```python
from build123d import *

# Parameters (mm, degrees)
SKETCH1_R           = 3.5
SKETCH1_R_2         = 1.5
SKETCH1_R_3         = 2.5
SKETCH1_W           = 2
SKETCH1_H           = 5
SKETCH1_W_2         = 5.5
SKETCH1_H_2         = 15.95
SKETCH1_H_3         = 14.5
BOSS_EXTRUDE1_DEPTH = 2
CUT_EXTRUDE_1_DEPTH = 10


with BuildPart() as part:
    # Sketch1 → Boss-Extrude1 (new body)
    with BuildSketch(Plane.XY):
        with BuildLine():
            Line((-25.65, 0), (25.65, 0))
            ThreePointArc((25.65, 0), (26.357106781, 0.292893219), (26.65, 1))
            Line((26.65, 1), (26.65, 99.754415082))
            ThreePointArc((26.65, 99.754415082), (25.980127019, 102.254415082), (24.15, 104.0845421))
            Line((24.15, 104.0845421), (7.5, 113.697424082))
            ThreePointArc((7.5, 113.697424082), (0, 115.707043026), (-7.5, 113.697424082))
            Line((-7.5, 113.697424082), (-24.15, 104.0845421))
            ThreePointArc((-24.15, 104.0845421), (-25.980127019, 102.254415082), (-26.65, 99.754415082))
            Line((-26.65, 99.754415082), (-26.65, 1))
            ThreePointArc((-26.65, 1), (-26.357106781, 0.292893219), (-25.65, 0))
        make_face()
        with Locations((0, 90)):
            Circle(SKETCH1_R, mode=Mode.SUBTRACT)
        with Locations((19.05, 66.1)):
            Circle(SKETCH1_R_2, mode=Mode.SUBTRACT)
        with Locations((-8.85, 66.1)):
            Circle(SKETCH1_R_2, mode=Mode.SUBTRACT)
        with Locations((-24.05, 15.3)):
            Circle(SKETCH1_R_2, mode=Mode.SUBTRACT)
        with Locations((24.15, 14)):
            Circle(SKETCH1_R_2, mode=Mode.SUBTRACT)
        with Locations((0, 34.3)):
            Circle(SKETCH1_R_3, mode=Mode.SUBTRACT)
        with Locations((4.5, 103.75)):
            Rectangle(SKETCH1_W, SKETCH1_H, mode=Mode.SUBTRACT)
        with Locations((9.55, 83.375)):
            Rectangle(SKETCH1_W_2, SKETCH1_H_2, mode=Mode.SUBTRACT)
        with Locations((20.15, 87)):
            Rectangle(SKETCH1_W, SKETCH1_H_3, mode=Mode.SUBTRACT)
        with Locations((4.5, 72.75)):
            Rectangle(SKETCH1_W, SKETCH1_H, mode=Mode.SUBTRACT)
        with Locations((-4.5, 72.75)):
            Rectangle(SKETCH1_W, SKETCH1_H, mode=Mode.SUBTRACT)
        with Locations((-20.15, 87)):
            Rectangle(SKETCH1_W, SKETCH1_H_3, mode=Mode.SUBTRACT)
        with Locations((-4.5, 103.75)):
            Rectangle(SKETCH1_W, SKETCH1_H, mode=Mode.SUBTRACT)
        with Locations((-13.15, 72.75)):
            Rectangle(SKETCH1_W, SKETCH1_H, mode=Mode.SUBTRACT)
        with Locations((-13.15, 87.75)):
            Rectangle(SKETCH1_W, SKETCH1_H, mode=Mode.SUBTRACT)
        Polygon((-20, 34.3), (-20, 36.05), (-7, 36.05), (-7, 34.3), (-7, 32.55), (-20, 32.55), align=None, mode=Mode.SUBTRACT)
        Polygon((-5.232050808, 39.362177826), (-15.732050808, 57.548711306), (-12.267949192, 59.548711306), (-1.767949192, 41.362177826), align=None, mode=Mode.SUBTRACT)
        Polygon((1.767949192, 41.362177826), (5.232050808, 39.362177826), (15.732050808, 57.548711306), (12.267949192, 59.548711306), align=None, mode=Mode.SUBTRACT)
        Polygon((7, 34.3), (7, 32.55), (20, 32.55), (20, 34.3), (20, 36.05), (7, 36.05), align=None, mode=Mode.SUBTRACT)
        Polygon((-1.767949192, 27.237822174), (-5.232050808, 29.237822174), (-15.732050808, 11.051288694), (-12.267949192, 9.051288694), align=None, mode=Mode.SUBTRACT)
        Polygon((15.732050808, 11.051288694), (12.267949192, 9.051288694), (1.767949192, 27.237822174), (5.232050808, 29.237822174), align=None, mode=Mode.SUBTRACT)
    extrude(amount=BOSS_EXTRUDE1_DEPTH)

    # 草图1 → 切除-拉伸1 (cut)
    with BuildSketch(Plane(origin=(0, 0, 0), x_dir=(-1, 0, 0), z_dir=(0, 0, -1))):
        Polygon((-26.65, 61.892241422), (26.65, 61.892241422), (26.65, 1), (26.65, 0), (-26.65, 0), align=None)
    extrude(amount=-CUT_EXTRUDE_1_DEPTH, mode=Mode.SUBTRACT)


solid = part.part
```
Source: CAD feature listing. Evaluate the final solid. Frame: model axes, mm. Give positions to 0.01 mm unless a question says otherwise; leave off trailing zeros. Write each loop counter-clockwise with the first axis right and the second up, starting at its lowest first coordinate (ties: lowest second). Pieces come first, ordered by that corner, then holes. Notation, with made-up numbers: (-14, -26.5) - (28, -26.5) arc R26 ccw to (28, -10.5) - close; hole circle Ø2 at (9, 24). An arc over 180 degrees is marked (long way). One line per item, written item: value. Start each with the question number.
Q1. Material intervals for probe 1 along X at (y, z) = (86, 0.75); probe 2 along X at (y, z) = (66.1, 0.55); probe 3 along X at (y, z) = (83, 0.6), sorted ascending. Write a range as from..to.
Q2. Section query A-A, the plane x = 0. Return the cut outline in (y, z).
Q3. Draft query along X for faces 1 (the face through (0, 61.892, 1)), 2 (the face through (20, 79.75, 1)). Return one class per face: +X half, -X half, draft (parallel to the pull), parting line (faces both ways), or undercut.
Q4. First-contact query: pin 1 Ø3.5 at (x, y) = (-8.85, 66.1) entering from -Z; pin 2 Ø0.6 at (y, z) = (104, 0.5) entering from +X; pin 3 Ø0.6 at (y, z) = (104, 1) entering from -X; pin 4 Ø1 at (x, z) = (-13.5, 1) entering from +Y. Flat tips, straight axial feed; report the tip coordinate or a pass-through.
Q5. Section query C-C, the plane y = 83.5. Return the cut outline in (x, z).
Q6. Section query D-D, the plane x = 11. Return the cut outline in (y, z), then the cut area to 3 significant figures.
Q7. Section query B-B, the plane y = 66.1. Return the cut outline in (x, z).
Answer:
1. probe 1: x = -26.65..-21.15, -19.15..-14.15, -12.15..6.8, 12.3..19.15, 21.15..26.65
1. probe 2: x = -26.65..-10.35, -7.35..17.55, 20.55..26.65
1. probe 3: x = -26.65..-21.15, -19.15..6.8, 12.3..19.15, 21.15..26.65
2. outline: (61.89, 0) - (86.5, 0) - (86.5, 2) - (61.89, 2) - close; (93.5, 0) - (115.71, 0) - (115.71, 2) - (93.5, 2) - close
3. face 1: draft
3. face 2: undercut
4. pin 1: stops at z = 0
4. pin 2: stops at x = 24.72
4. pin 3: stops at x = -24.72
4. pin 4: stops at y = 110.52
5. outline: (-26.65, 0) - (-21.15, 0) - (-21.15, 2) - (-26.65, 2) - close; (-19.15, 0) - (6.8, 0) - (6.8, 2) - (-19.15, 2) - close; (12.3, 0) - (19.15, 0) - (19.15, 2) - (12.3, 2) - close; (21.15, 0) - (26.65, 0) - (26.65, 2) - (21.15, 2) - close
6. outline: (61.89, 0) - (75.4, 0) - (75.4, 2) - (61.89, 2) - close; (91.35, 0) - (111.68, 0) - (111.68, 2) - (91.35, 2) - close
6. area: 67.7 mm2
7. outline: (-26.65, 0) - (-10.35, 0) - (-10.35, 2) - (-26.65, 2) - close; (-7.35, 0) - (17.55, 0) - (17.55, 2) - (-7.35, 2) - close; (20.55, 0) - (26.65, 0) - (26.65, 2) - (20.55, 2) - close
